```python
from build123d import *

# Parameters (mm, degrees)
SKETCH1_R           = 6
BOSS_EXTRUDE1_DEPTH = 3
SKETCH2_W           = 11
SKETCH2_H           = 15
BOSS_EXTRUDE2_DEPTH = 2
SKETCH3_W           = 6
SKETCH3_H           = 6
CUT_EXTRUDE1_DEPTH  = 12.113055385
CHAMFER1_SIZE       = 0.5


with BuildPart() as part:
    # Sketch1 → Boss-Extrude1 (new body)
    with BuildSketch(Plane.XY):
        Circle(SKETCH1_R)
    extrude(amount=BOSS_EXTRUDE1_DEPTH)

    # Sketch2 → Boss-Extrude2 (add)
    with BuildSketch(Plane.XY.offset(3)):
        with Locations((1, 0)):
            Rectangle(SKETCH2_W, SKETCH2_H)
    extrude(amount=BOSS_EXTRUDE2_DEPTH)

    # Sketch3 → Cut-Extrude1 (cut, through all)
    with BuildSketch(Plane(origin=(0, 0, 0), x_dir=(-1, 0, 0), z_dir=(0, 0, -1))):
        Rectangle(SKETCH3_W, SKETCH3_H)
    extrude(amount=-CUT_EXTRUDE1_DEPTH, mode=Mode.SUBTRACT)

    # Chamfer1
    chamfer1_edges = [part.edges().sort_by_distance(p)[0] for p in [
        (3, 0, 5),
        (0, 3, 5),
        (-3, 0, 5),
        (0, -3, 5),
    ]]
    chamfer(chamfer1_edges, length=CHAMFER1_SIZE)


solid = part.part
```
The listing builds one solid part. Answer for the finished solid, in the listing's coordinates (mm). A direction names the side the tool comes from. Give positions to 0.01 mm unless a question says otherwise; leave off trailing zeros. Loops run counter-clockwise (first coordinate to the right, second up) from the corner with the lowest first, then second, coordinate; pieces in that order, holes last. Notation, with made-up numbers: M 13.25,38.5 L 50.25,38.5 A7 cw 50.25,43.5 Z; hole C 81.25,28.5 d2. An arc over 180 degrees is marked long. One line per item, written item: value.
1. For faces 5 (the face through (-5, 0, 3)), 6 (the face through (0, 3, 2)), 7 (the face through (5, 0, 5)), 8 (the face through (-6, 0, 1)), 9 (the face through (0, -4, 0)), determine the directions among +Z, -Z, +X, -X, +Y, -Y from which every point of the face is accessible in a straight line to the end or side of a thin tool.
Found:
face 5: +Z, -X, +Y, -Y
face 6: +Z, -Z
face 7: +Z, +X, -X, +Y, -Y
face 8: -Z
face 9: -Z, +X, -X, +Y, -Y
2. Each of these flat-tipped pins is pushed along its axis until it touches: P1, Ø2, axis at y = 1, z = 1.5, coming from the +X side; P2, Ø1.3, axis at y = 1, z = 2.5, coming from the -X side. Where does it stop, or does it pass through?
Found:
P1: x = 6
P2: x = -5.99
3. Find the intervals of material crossed by probe 1 along Y at (x, z) = (0, 3.05); probe 2 along X at (y, z) = (0, 2.45); probe 3 along Z at (x, y) = (4.5, -4.75), in increasing order.
Found:
probe 1: -7.5 to -3, 3 to 7.5
probe 2: -6 to -3, 3 to 6
probe 3: 3 to 5
4. Section D-D on z = 0.7 is taken. Determine the outline of the cut face in (x, y).
Found:
outline: C 0,0 d12; hole M -3,-3 L 3,-3 L 3,3 L -3,3 Z
5. Section A-A on x = 0 is taken. Determine the outline of the cut face in (y, z).
Found:
outline: M -7.5,3 L -6,3 L -6,0 L -3,0 L -3,4.5 L -3.5,5 L -7.5,5 Z; M 3,0 L 6,0 L 6,3 L 7.5,3 L 7.5,5 L 3.5,5 L 3,4.5 Z
6. Section C-C on z = 3.65 is taken. Determine the outline of the cut face in (x, y), plus the area to 3 significant figures.
Found:
outline: M -4.5,-7.5 L 6.5,-7.5 L 6.5,7.5 L -4.5,7.5 Z; hole M -3,-3 L 3,-3 L 3,3 L -3,3 Z
area: 129 mm^2
7. Section B-B on y = 0 is taken. Determine the outline of the cut face in (x, z).
Found:
outline: M -6,0 L -3,0 L -3,4.5 L -3.5,5 L -4.5,5 L -4.5,3 L -6,3 Z; M 3,0 L 6,0 L 6,3 L 6.5,3 L 6.5,5 L 3.5,5 L 3,4.5 Z
8. For a pull along Y with two mould halves and no side action, classify faces 1 (the face through (1, 7.5, 4)), 2 (the face through (0, -3, 2)), 3 (the face through (1, -7.5, 4)), 4 (the face through (-4.5, 0, 4)) as pulls with the +Y half, pulls with the -Y half, needs draft (parallel to the pull), parting line crosses it, or undercut.
Found:
face 1: pulls with the +Y half
face 2: undercut
face 3: pulls with the -Y half
face 4: needs draft
